Design review of the part built by this model. Coordinates are the model's own, in mm. Face numbers are marked on the shaded views. A direction names the side the tool comes from. Coordinates: 2 decimals unless noted, no trailing zeros. Loops run counter-clockwise (first coordinate to the right, second up) from the corner with the lowest first, then second, coordinate; pieces in that order, holes last. Notation, with made-up numbers: (-34, 12.25) - (8, 12.25) arc R20 ccw to (8, 19.25) - close; hole circle Ø7 at (-1, -19.5). An arc over 180 degrees is marked (long way). One line per question, with ' | ' between items.
from build123d import *

# Parameters (mm, degrees)
SKETCH2_W           = 200
SKETCH2_H           = 96.666666667
BOSS_EXTRUDE2_DEPTH = 60
FILLET12_R          = 48.333333
SKETCH6_R           = 12.5
CUT_EXTRUDE3_DEPTH  = 61
SKETCH8_W           = 60
SKETCH8_H           = 35
BOSS_EXTRUDE3_DEPTH = 50
SKETCH10_R          = 10
CUT_EXTRUDE4_DEPTH  = 50


with BuildPart() as part:
    # Sketch2 → Boss-Extrude2 (new body)
    with BuildSketch(Plane.XY):
        with Locations((100, -48.333333334)):
            Rectangle(SKETCH2_W, SKETCH2_H)
    extrude(amount=-BOSS_EXTRUDE2_DEPTH)

    # Fillet12
    fillet12_edges = [part.edges().sort_by_distance(p)[0] for p in [
        (200, 0, -30),
        (200, -96.666666667, -30),
    ]]
    fillet(fillet12_edges, radius=FILLET12_R)

    # Sketch6 → Cut-Extrude3 (cut, through all)
    with BuildSketch(Plane(origin=(0, 0, -60), x_dir=(-1, 0, 0), z_dir=(0, 0, -1))):
        with Locations((-151.666666667, -48.333333333)):
            Circle(SKETCH6_R)
    extrude(amount=-CUT_EXTRUDE3_DEPTH, mode=Mode.SUBTRACT)

    # Sketch8 → Boss-Extrude3 (add)
    with BuildSketch(Plane.ZY):
        with Locations((-30, -17.5)):
            Rectangle(SKETCH8_W, SKETCH8_H)
    extrude(amount=BOSS_EXTRUDE3_DEPTH)

    # Sketch10 → Cut-Extrude4 (cut)
    with BuildSketch(Plane(origin=(0, 0, 0), x_dir=(1, 0, 0), z_dir=(0, 1, 0))):
        with Locations((-30, 30)):
            Circle(SKETCH10_R)
    extrude(amount=-CUT_EXTRUDE4_DEPTH, mode=Mode.SUBTRACT)


solid = part.part
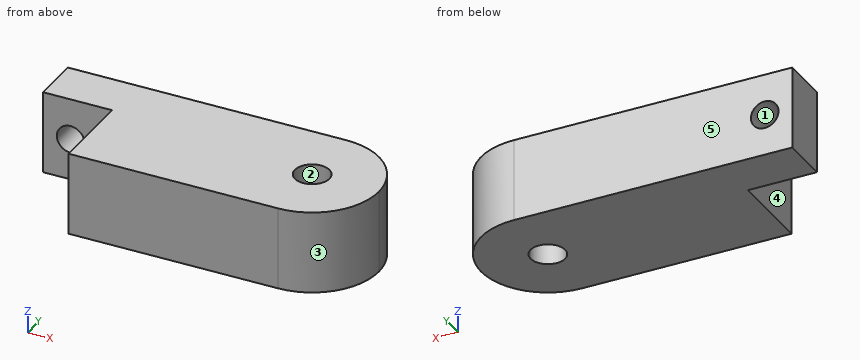
Q1. Take a section at C-C (z = -55). Give the boundary of the cut face in (x, y).
Returned:
outline: (-50, -35) - (0, -35) - (0, -96.67) - (151.67, -96.67) arc R48.33 ccw to (151.67, 0) - (-50, 0) - close; hole circle Ø25 at (151.67, -48.33)
Q2. Take a section at B-B (x = -30). Give the boundary of the cut face in (y, z).
Returned:
outline: (-35, -60) - (0, -60) - (0, -40) - (-35, -40) - close; (-35, -20) - (0, -20) - (0, 0) - (-35, 0) - close
Q3. To check wall thickness, follow line 1 along Y through (x, z) = (151, -45); line 2 along Z through (x, y) = (-30, -20); line 3 along Y through (x, z) = (-32.5, -49). State the ranges of each line that lie inside material, in increasing order.
Returned:
line 1: y = -96.67 to -60.82, -35.85 to 0 | line 2: z = -60 to -40, -20 to 0 | line 3: y = -35 to 0
Q4. Take a section at A-A (z = -30). Give the boundary of the cut face in (x, y).
Returned:
outline: (-50, -35) - (-40, -35) - (-40, 0) - (-50, 0) - close; (-20, -35) - (0, -35) - (0, -96.67) - (151.67, -96.67) arc R48.33 ccw to (151.67, 0) - (-20, 0) - close; hole circle Ø25 at (151.67, -48.33)
Q5. Tool access review of the marked faces 4 and 5: name each direction out of +Z, -Z, +X, -X, +Y, -Y from which nothing blocks a thin tool from reaching the whole face with its end or side.
Returned:
face 4: +Z, -Z, -X, -Y | face 5: +Z, -Z, +X, -X, +Y
Q6. Draft analysis for pull direction Y (two halves, no side actions). For the marked faces 1, 2 and 3, state which applies: +Y half, -Y half, draft (parallel to the pull), parting line (faces both ways), or undercut.
Returned:
face 1: draft | face 2: undercut | face 3: -Y half
Q7. For pin 1 (10 mm diameter, centred on y = -75, z = -51.5, fed in from -X); pin 2 (2 mm diameter, centred on x = 51, y = -70.5, fed in from +Z); pin 3 (16 mm diameter, centred on x = -30, z = -30, fed in from -Y); pin 4 (5 mm diameter, centred on x = 164.5, z = -12, fed in from +Y), all flat-tipped, find the tip position at first contact; note any pin that passes through.
Returned:
pin 1: stops at x = 0 | pin 2: stops at z = 0 | pin 3: passes through | pin 4: stops at y = -1.12
Q8. Take a section at D-D (y = -52). Give the boundary of the cut face in (x, z).
Returned:
outline: (0, -60) - (139.72, -60) - (139.72, 0) - (0, 0) - close; (163.62, -60) - (199.86, -60) - (199.86, 0) - (163.62, 0) - close
